Design review of the part built by this model. Coordinates are the model's own, in mm. A direction names the side the tool comes from. Give positions to 0.01 mm unless a question says otherwise; leave off trailing zeros. Write each loop counter-clockwise with the first axis right and the second up, starting at its lowest first coordinate (ties: lowest second). Pieces come first, ordered by that corner, then holes.
```python
from build123d import *

# Parameters (mm, degrees)
SKETCH1_R                    = 20
BOSS_EXTRUDE1_DEPTH          = 15
SKETCH2_R                    = 1.5
CUT_EXTRUDE1_DEPTH           = 20
SKETCH3_R                    = 2.5
CUT_EXTRUDE2_DEPTH           = 2.5
CUT_EXTRUDE2_DRAFT           = -20.5
CUT_EXTRUDE2_PROFILE_2_DEPTH = 2.5
CUT_EXTRUDE2_PROFILE_2_DRAFT = -20.5
CUT_EXTRUDE2_PROFILE_3_DEPTH = 2.5
CUT_EXTRUDE2_PROFILE_3_DRAFT = -20.5
CUT_EXTRUDE2_PROFILE_4_DEPTH = 2.5
CUT_EXTRUDE2_PROFILE_4_DRAFT = -20.5
SKETCH4_R                    = 14
CUT_EXTRUDE3_DEPTH           = 12
SKETCH5_R                    = 11
CUT_EXTRUDE4_DEPTH           = 12


with BuildPart() as part:
    # Sketch1 → Boss-Extrude1 (new body)
    with BuildSketch(Plane(origin=(0, 0, 0), x_dir=(1, 0, 0), z_dir=(0, 1, 0))):
        with Locations(Location((0, 0, 0), (0, 0, 270))):
            Circle(SKETCH1_R)
    extrude(amount=BOSS_EXTRUDE1_DEPTH)

    # Sketch2 → Cut-Extrude1 (cut)
    with BuildSketch(Plane(origin=(0, 0, 0), x_dir=(-1, 0, 0), z_dir=(0, -1, 0))):
        with Locations(Location((0, -17, 0), (0, 0, 90))):
            Circle(SKETCH2_R)
        with Locations(Location((-17, 0, 0), (0, 0, 90))):
            Circle(SKETCH2_R)
        with Locations(Location((0, 17, 0), (0, 0, 90))):
            Circle(SKETCH2_R)
        with Locations(Location((17, 0, 0), (0, 0, 90))):
            Circle(SKETCH2_R)
    extrude(amount=-CUT_EXTRUDE1_DEPTH, mode=Mode.SUBTRACT)


with BuildPart() as cut_extrude2_tool:
    # Sketch3 → Cut-Extrude2 (with draft: the straight prism first)
    with BuildSketch(Plane(origin=(0, 15, 0), x_dir=(1, 0, 0), z_dir=(0, 1, 0))):
        with Locations((0, 17)):
            Circle(SKETCH3_R)
    extrude(amount=-CUT_EXTRUDE2_DEPTH)
    # Cut-Extrude2: the draft: its side faces are tilted about the plane it starts from
    cut_extrude2_sides = [cut_extrude2_tool.faces().sort_by_distance(p)[0] for p in [
        (-2.5, 13.75, -17),
    ]]
    draft(cut_extrude2_sides, Plane(origin=(0, 15, 0), x_dir=(1, 0, 0), z_dir=(0, 1, 0)), CUT_EXTRUDE2_DRAFT)


with BuildPart() as part_1:
    add(part.part)

    # Cut-Extrude2: cut by cut_extrude2_tool
    add(cut_extrude2_tool.part, mode=Mode.SUBTRACT)


with BuildPart() as cut_extrude2_profile_2_tool:
    # Sketch3 → Cut-Extrude2 profile 2 (with draft: the straight prism first)
    with BuildSketch(Plane(origin=(0, 15, 0), x_dir=(1, 0, 0), z_dir=(0, 1, 0))):
        with Locations((17, 0)):
            Circle(SKETCH3_R)
    extrude(amount=-CUT_EXTRUDE2_PROFILE_2_DEPTH)
    # Cut-Extrude2 profile 2: the draft: its side faces are tilted about the plane it starts from
    cut_extrude2_profile_2_sides = [cut_extrude2_profile_2_tool.faces().sort_by_distance(p)[0] for p in [
        (14.5, 13.75, 0),
    ]]
    draft(cut_extrude2_profile_2_sides, Plane(origin=(0, 15, 0), x_dir=(1, 0, 0), z_dir=(0, 1, 0)), CUT_EXTRUDE2_PROFILE_2_DRAFT)


with BuildPart() as part_2:
    add(part_1.part)

    # Cut-Extrude2 profile 2: cut by cut_extrude2_profile_2_tool
    add(cut_extrude2_profile_2_tool.part, mode=Mode.SUBTRACT)


with BuildPart() as cut_extrude2_profile_3_tool:
    # Sketch3 → Cut-Extrude2 profile 3 (with draft: the straight prism first)
    with BuildSketch(Plane(origin=(0, 15, 0), x_dir=(1, 0, 0), z_dir=(0, 1, 0))):
        with Locations((0, -17)):
            Circle(SKETCH3_R)
    extrude(amount=-CUT_EXTRUDE2_PROFILE_3_DEPTH)
    # Cut-Extrude2 profile 3: the draft: its side faces are tilted about the plane it starts from
    cut_extrude2_profile_3_sides = [cut_extrude2_profile_3_tool.faces().sort_by_distance(p)[0] for p in [
        (-2.5, 13.75, 17),
    ]]
    draft(cut_extrude2_profile_3_sides, Plane(origin=(0, 15, 0), x_dir=(1, 0, 0), z_dir=(0, 1, 0)), CUT_EXTRUDE2_PROFILE_3_DRAFT)


with BuildPart() as part_3:
    add(part_2.part)

    # Cut-Extrude2 profile 3: cut by cut_extrude2_profile_3_tool
    add(cut_extrude2_profile_3_tool.part, mode=Mode.SUBTRACT)


with BuildPart() as cut_extrude2_profile_4_tool:
    # Sketch3 → Cut-Extrude2 profile 4 (with draft: the straight prism first)
    with BuildSketch(Plane(origin=(0, 15, 0), x_dir=(1, 0, 0), z_dir=(0, 1, 0))):
        with Locations((-17, 0)):
            Circle(SKETCH3_R)
    extrude(amount=-CUT_EXTRUDE2_PROFILE_4_DEPTH)
    # Cut-Extrude2 profile 4: the draft: its side faces are tilted about the plane it starts from
    cut_extrude2_profile_4_sides = [cut_extrude2_profile_4_tool.faces().sort_by_distance(p)[0] for p in [
        (-19.5, 13.75, 0),
    ]]
    draft(cut_extrude2_profile_4_sides, Plane(origin=(0, 15, 0), x_dir=(1, 0, 0), z_dir=(0, 1, 0)), CUT_EXTRUDE2_PROFILE_4_DRAFT)


with BuildPart() as part_4:
    add(part_3.part)

    # Cut-Extrude2 profile 4: cut by cut_extrude2_profile_4_tool
    add(cut_extrude2_profile_4_tool.part, mode=Mode.SUBTRACT)

    # Sketch4 → Cut-Extrude3 (cut)
    with BuildSketch(Plane.XZ):
        with Locations(Location((0, 0, 0), (0, 0, 270))):
            Circle(SKETCH4_R)
    extrude(amount=-CUT_EXTRUDE3_DEPTH, mode=Mode.SUBTRACT)

    # Sketch5 → Cut-Extrude4 (cut)
    with BuildSketch(Plane(origin=(0, 15, 0), x_dir=(1, 0, 0), z_dir=(0, 1, 0))):
        with Locations(Location((0, 0, 0), (0, 0, 270))):
            Circle(SKETCH5_R)
    extrude(amount=-CUT_EXTRUDE4_DEPTH, mode=Mode.SUBTRACT)


solid = part_4.part
```
(1) Consider section A-A, the plane z = 0. Give the boundary of the cut face in (x, y), then the cut area to 3 significant figures.
Resolved:
outline: (-20, 0) - (-18.5, 0) - (-18.5, 12.5) - (-18.57, 12.5) - (-19.5, 15) - (-20, 15) - close; (-15.5, 0) - (-14, 0) - (-14, 12) - (-11, 12) - (-11, 15) - (-14.5, 15) - (-15.43, 12.5) - (-15.5, 12.5) - close; (11, 12) - (14, 12) - (14, 0) - (15.5, 0) - (15.5, 12.5) - (15.43, 12.5) - (14.5, 15) - (11, 15) - close; (18.5, 0) - (20, 0) - (20, 15) - (19.5, 15) - (18.57, 12.5) - (18.5, 12.5) - close
area: 103 mm2
(2) Mouldability with a two-part tool opening along Z and no side actions: class faces 3 (the face through (12, 0, -8)), 4 (the face through (-19.524, 7.395, -4.336)), 5 (the face through (18.265, 6.162, -0.806)) as pulls with the +Z half, pulls with the -Z half, needs draft (parallel to the pull), parting line crosses it, or undercut.
Resolved:
face 3: needs draft
face 4: parting line crosses it
face 5: undercut
(3) Tool access review of faces 1 (the face through (-0.397, 13.212, -15.212)), 2 (the face through (-13.67, 5.92, 3.03)): name each direction out of +Z, -Z, +X, -X, +Y, -Y from which nothing blocks a thin tool from reaching the whole face with its end or side.
Resolved:
face 1: +Y
face 2: -Y
(4) Consider section C-C, the plane x = 17. Give the boundary of the cut face in (y, z).
Resolved:
outline: (0, -10.54) - (15, -10.54) - (15, -2.5) - (12.5, -1.57) - (12.5, -1.5) - (0, -1.5) - close; (0, 1.5) - (12.5, 1.5) - (12.5, 1.57) - (15, 2.5) - (15, 10.54) - (0, 10.54) - close
(5) To check wall thickness, follow L1, parallel to X at y = 3.75, z = 0; L2, parallel to Z at x = 17, y = 13.25; L3, parallel to X at y = 7.25, z = -17. State the ranges of each line that lie inside material, in increasing order.
Resolved:
L1: x = -20 to -18.5, -15.5 to -14, 14 to 15.5, 18.5 to 20
L2: z = -10.54 to -1.85, 1.85 to 10.54
L3: x = -10.54 to -1.5, 1.5 to 10.54
(6) Consider section B-B, the plane x = 0. Give the boundary of the cut face in (y, z), then the cut area to 3 significant figures.
Resolved:
outline: (0, -20) - (15, -20) - (15, -19.5) - (12.5, -18.57) - (12.5, -18.5) - (0, -18.5) - close; (0, -15.5) - (12.5, -15.5) - (12.5, -15.43) - (15, -14.5) - (15, -11) - (12, -11) - (12, -14) - (0, -14) - close; (0, 14) - (12, 14) - (12, 11) - (15, 11) - (15, 14.5) - (12.5, 15.43) - (12.5, 15.5) - (0, 15.5) - close; (0, 18.5) - (12.5, 18.5) - (12.5, 18.57) - (15, 19.5) - (15, 20) - (0, 20) - close
area: 103 mm2
(7) Consider section D-D, the plane z = -5.5. Give the boundary of the cut face in (x, y).
Resolved:
outline: (-19.23, 0) - (-12.87, 0) - (-12.87, 12) - (-9.53, 12) - (-9.53, 15) - (-19.23, 15) - close; (9.53, 12) - (12.87, 12) - (12.87, 0) - (19.23, 0) - (19.23, 15) - (9.53, 15) - close
(8) Clearance check with flat-ended pins moving along their axes: P1, Ø8, axis at y = 7, z = -2.5, coming from the -X side; P2, Ø2, axis at x = -15, y = 13, coming from the -Z side; P3, Ø4, axis at x = -3.5, y = 2, coming from the -Z side. State where each tip first meets the part, or that it passes through.
Resolved:
P1: stops at x = -20
P2: stops at z = -14.28
P3: stops at z = -19.94
